Study the drawing (mm; zero at the part's minimum x, y, z) and answer. A direction names the side the tool comes from. Round coordinates to 2 decimals unless told otherwise and drop trailing zeros. Loops run counter-clockwise (first coordinate to the right, second up) from the corner with the lowest first, then second, coordinate; pieces in that order, holes last. Notation, with made-up numbers: (16.5, 58) -> (51.5, 58) arc R5 ccw to (51.5, 62) -> close; hole circle Ø7 at (26, 22.5). An arc over 180 degrees is marked (long way). Use one line per item in the form item = value.
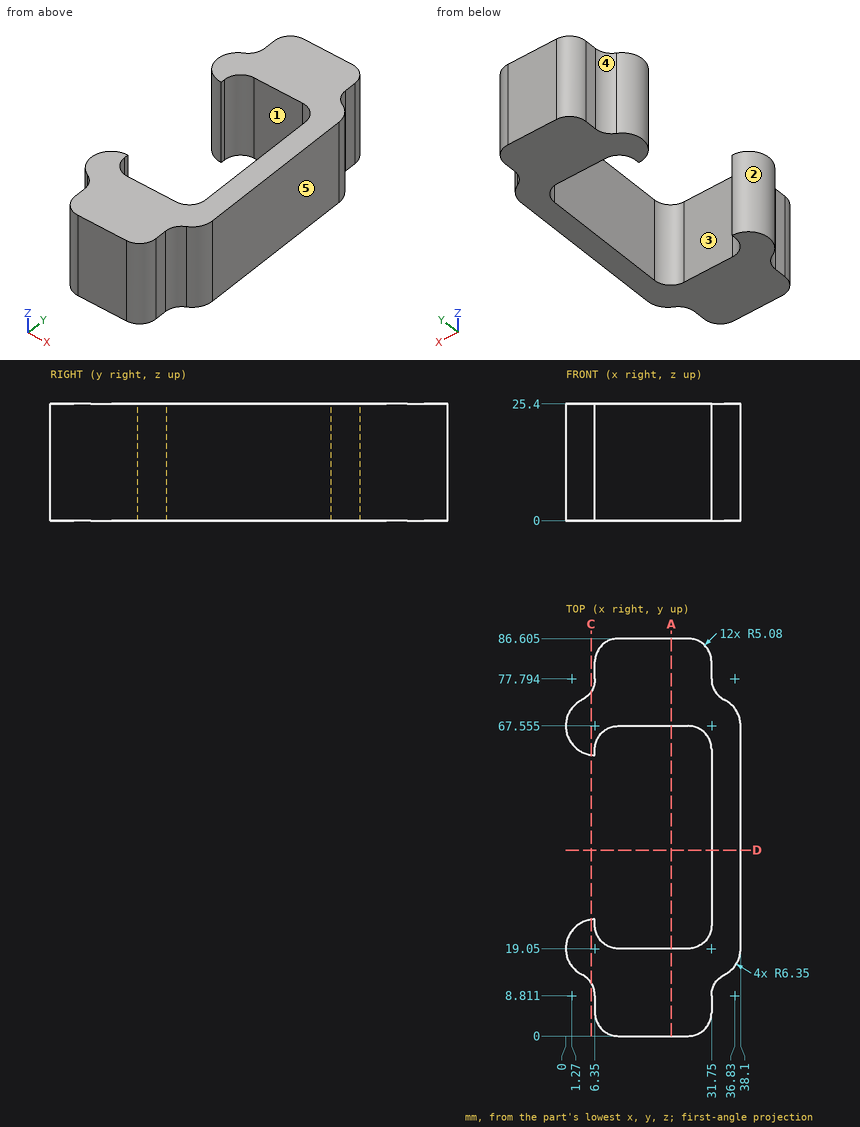
(1) Find section A-A, the plane x = 23. Write down the section's boundary in (y, z) (3 decimals), then the cut area to 3 significant figures.
Completed:
outline = (0, 0) -> (19.05, 0) -> (19.05, 25.4) -> (0, 25.4) -> close; (67.555, 0) -> (86.605, 0) -> (86.605, 25.4) -> (67.555, 25.4) -> close
area = 968 mm2
(2) For a pull along X with two mould halves and no side action, classify the marked faces 3, 4 and 5 as +X half, -X half, draft (parallel to the pull), parting line (faces both ways), or undercut.
Completed:
face_3 = undercut
face_4 = -X half
face_5 = +X half
(3) Find section D-D, the plane y = 40.5. Write down the section's boundary in (x, z).
Completed:
outline = (31.75, 0) -> (38.1, 0) -> (38.1, 25.4) -> (31.75, 25.4) -> close
(4) Consider L1, parallel to Y at x = 27, z = 22; L2, parallel to Y at x = 20, z = 14 (3 decimals); L3, parallel to X at y = 47.5, z = 7.75. Determine where each line is inside the solid, lowest interval first.
Completed:
L1 = 0.01 to 19.06, 67.54 to 86.59
L2 = 0 to 19.05, 67.555 to 86.605
L3 = 31.75 to 38.1
(5) For the marked faces 1 and 2, determine the directions among +Z, -Z, +X, -X, +Y, -Y from which every point of the face is accessible in a straight line to the end or side of a thin tool.
Completed:
face_1 = +Z, -Z
face_2 = +Z, -Z, -X
(6) Find section C-C, the plane x = 5.5. Write down the section's boundary in (y, z).
Completed:
outline = (11.62, 0) -> (25.34, 0) -> (25.34, 25.4) -> (11.62, 25.4) -> close; (61.26, 0) -> (74.98, 0) -> (74.98, 25.4) -> (61.26, 25.4) -> close
(7) Given P1, Ø3, axis at y = 6.5, z = 18, coming from the +X side; P2, Ø3, axis at x = 13.5, z = 22.5, coming from the -Y side; P3, Ø8, axis at x = 6.5, z = 19, coming from the +Y side; P4, Ø12.5, axis at y = 49, z = 15, coming from the -X side, each flat-ended and moving along its own axis, determine where each tip first touches the part or whether it passes through.
Completed:
P1 = 31.75
P2 = 0
P3 = 86.52
P4 = 31.75
